Read the model definition and answer for the solid it produces. Units are mm, in the model's axes. Round coordinates to 2 decimals unless told otherwise and drop trailing zeros. Write each loop counter-clockwise with the first axis right and the second up, starting at its lowest first coordinate (ties: lowest second). Pieces come first, ordered by that corner, then holes. Notation, with made-up numbers: M -26.5,83 L -7.5,83 A20 ccw -7.5,90 Z; hole C -35,25 d6. An arc over 180 degrees is marked long. Use one line per item in the form item = value. Start each with the question number.
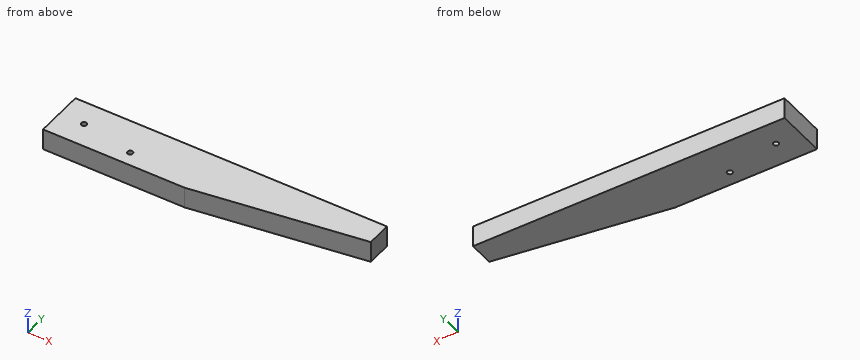
```python
from build123d import *

# Parameters (mm, degrees)
SKETCH1_W                        = 558.8
SKETCH1_H                        = 88.9
BOSS_EXTRUDE1_DEPTH              = 38.1
CUT_EXTRUDE1_DEPTH               = 568.108684469
F_3_8_0_375_DIAMETER_HOLE1_D     = 9.525
F_3_8_0_375_DIAMETER_HOLE1_DEPTH = 76.2
F_3_8_0_375_DIAMETER_HOLE1_TIP   = 2.861598698
SKETCH8_R                        = 4.7625
CUT_EXTRUDE2_DEPTH               = 568.108684469


with BuildPart() as part:
    # Sketch1 → Boss-Extrude1 (new body)
    with BuildSketch(Plane.XY):
        with Locations((279.4, 44.45)):
            Rectangle(SKETCH1_W, SKETCH1_H)
    extrude(amount=BOSS_EXTRUDE1_DEPTH)

    # Sketch2 → Cut-Extrude1 (cut, through all)
    with BuildSketch(Plane.XY.offset(38.1)):
        Polygon((558.8, 44.45), (254, 0), (558.8, 0), align=None)
    extrude(amount=-CUT_EXTRUDE1_DEPTH, mode=Mode.SUBTRACT)

    # 3/8 (0.375) Diameter Hole1
    with Locations(Plane.XY.offset(38.1)):
        with Locations((44.45, 44.45)):
            Hole(F_3_8_0_375_DIAMETER_HOLE1_D / 2, depth=F_3_8_0_375_DIAMETER_HOLE1_DEPTH)
            with Locations((0, 0, -(F_3_8_0_375_DIAMETER_HOLE1_DEPTH + F_3_8_0_375_DIAMETER_HOLE1_TIP / 2))):  # 118° drill point
                Cone(0, F_3_8_0_375_DIAMETER_HOLE1_D / 2, F_3_8_0_375_DIAMETER_HOLE1_TIP, mode=Mode.SUBTRACT)

    # Sketch8 → Cut-Extrude2 (cut, through all)
    with BuildSketch(Plane.XY.offset(38.1)):
        with Locations((139.7, 25.4)):
            Circle(SKETCH8_R)
    extrude(amount=-CUT_EXTRUDE2_DEPTH, mode=Mode.SUBTRACT)


solid = part.part
```
Q1. Find section B-B on y = 15. Write down the section's boundary in (x, z), and give its area (3 significant figures).
Q2. Find section A-A on x = 139.7. Write down the section's boundary in (y, z), and give its area (3 significant figures).
Q3. Find section C-C on x = 459.5. Write down the section's boundary in (y, z), and give its area (3 significant figures).
Q4. Each of these flat-tipped pins is pushed along its axis until it touches: pin 1 Ø5 at (x, z) = (352, 24.5) entering from -Y; pin 2 Ø8 at (x, z) = (388.5, 5.5) entering from -Y. Where does it stop, or does it pass through?
Q5. Straight lines are drawn through the part: line 1 (Y direction, x = 44.45, z = 14.5); line 2 (Y direction, x = 282.5, z = 16.5); line 3 (Y direction, x = 281, z = 18). For each, find the intervals that lie inside material, in ascending order. Write a range as [from, to].
Response:
q1.outline = M 0,0 L 356.86,0 L 356.86,38.1 L 0,38.1 Z
q1.area = 13,600 mm²
q2.outline = M 0,0 L 20.64,0 L 20.64,38.1 L 0,38.1 Z; M 30.16,0 L 88.9,0 L 88.9,38.1 L 30.16,38.1 Z
q2.area = 3,020 mm²
q3.outline = M 29.97,0 L 88.9,0 L 88.9,38.1 L 29.97,38.1 Z
q3.area = 2,250 mm²
q4.pin_1 = 13.93
q4.pin_2 = 19.03
q5.line_1 = [0, 39.69], [49.21, 88.9]
q5.line_2 = [4.16, 88.9]
q5.line_3 = [3.94, 88.9]
